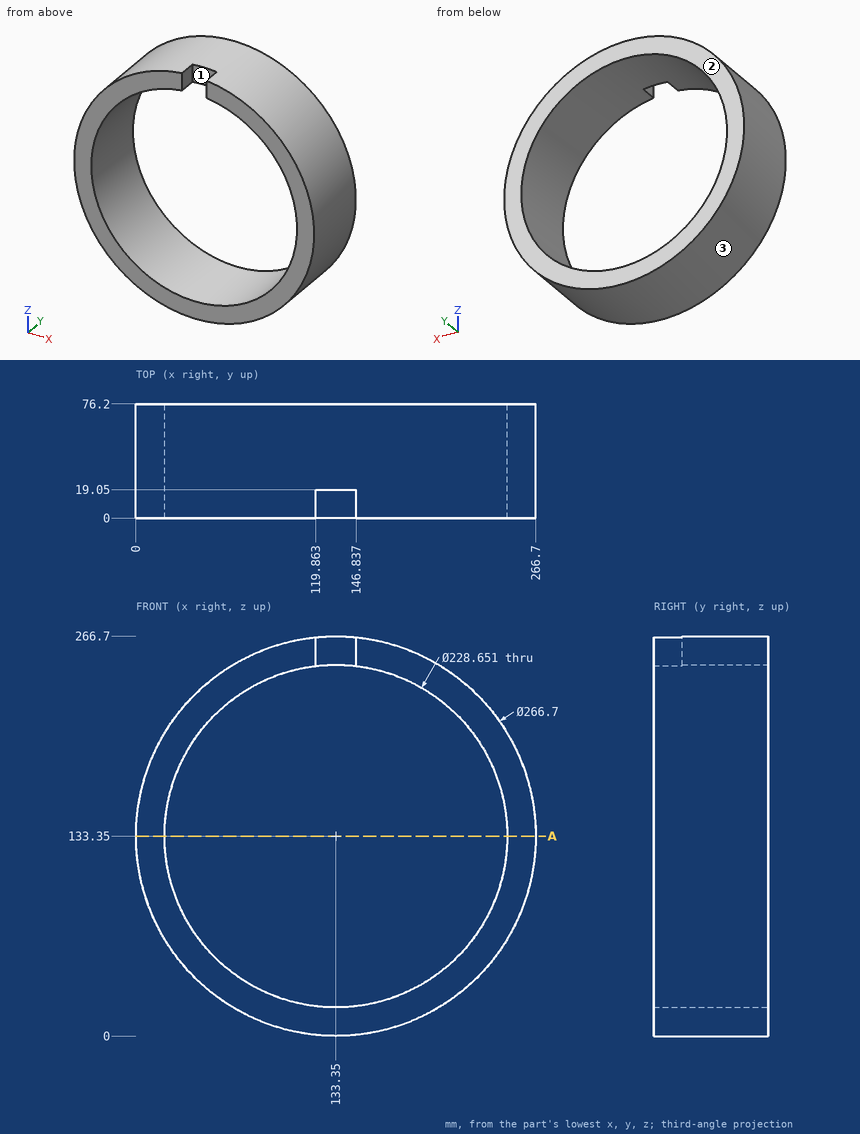
Part print with two shaded views. Sizes in mm from the minimum x, y, z corner. Coordinates: 2 decimals unless noted, no trailing zeros. Write each loop counter-clockwise with the first axis right and the second up, starting at its lowest first coordinate (ties: lowest second). Pieces come first, ordered by that corner, then holes.
(1) Mould opens along X. For the marked faces 1, 2 and 3 say: pulls with the +X half, pulls with the -X half, needs draft (parallel to the pull), parting line crosses it, or undercut.
(2) Drill centre lines: line 1 (X direction, y = 55, z = 133) (1 decimal); line 2 (Z direction, x = 190, y = 66.5). Where is each one in solid material? Low to high.
(3) Pin check, flat tips, straight feed: pin 1 Ø2 at (x, y) = (188, 49) entering from -Z; pin 2 Ø9.5 at (y, z) = (10, 254) entering from -X; pin 3 Ø2 at (x, y) = (75, 57) entering from +Z. Stop position of each tip, or through.
(4) Cut at A-A on z = 133.35. List the corners of the cut face in (x, y) (1 decimal), and give its area (3 significant figures).
Working result:
1. face 1: undercut
1. face 2: needs draft
1. face 3: parting line crosses it
2. line 1: x = 0 to 19, 247.7 to 266.7
2. line 2: z = 12.63 to 34.05, 232.65 to 254.07
3. pin 1: stops at z = 11.27
3. pin 2: stops at x = 67.4
3. pin 3: stops at z = 253.74
4. outline: (0, 0) - (19, 0) - (19, 76.2) - (0, 76.2) - close; (247.7, 0) - (266.7, 0) - (266.7, 76.2) - (247.7, 76.2) - close
4. area: 2,900 mm2
